```python
from build123d import *

# Parameters (mm, degrees)
SKETCH_R      = 6
SKETCH_R_2    = 3.4
PAD_DEPTH     = 8
SKETCH001_R   = 8.8
SKETCH001_R_2 = 3.4
PAD001_DEPTH  = 1
SKETCH002_R   = 4.2
SKETCH002_R_2 = 3.4
PAD002_DEPTH  = 8
FILLET_R      = 4.4


with BuildPart() as part:
    # Sketch → Pad (new body)
    with BuildSketch(Plane.XY):
        Circle(SKETCH_R)
        Circle(SKETCH_R_2, mode=Mode.SUBTRACT)
    extrude(amount=PAD_DEPTH)

    # Sketch001 → Pad001 (new body)
    with BuildSketch(Plane.XY.offset(8)):
        Circle(SKETCH001_R)
        Circle(SKETCH001_R_2, mode=Mode.SUBTRACT)
    extrude(amount=PAD001_DEPTH)

    # Sketch002 → Pad002 (new body)
    with BuildSketch(Plane.XY.offset(9)):
        Circle(SKETCH002_R)
        Circle(SKETCH002_R_2, mode=Mode.SUBTRACT)
    extrude(amount=PAD002_DEPTH)

    # Fillet
    fillet_edges = [part.edges().sort_by_distance(p)[0] for p in [
        (-4.2, 0, 9),
    ]]
    fillet(fillet_edges, radius=FILLET_R)


solid = part.part
```
Check sheet for the modelled part. Datum: model origin and axes. Units: mm. A direction names the side the tool comes from. Coordinates: 2 decimals unless noted, no trailing zeros. Loops run counter-clockwise (first coordinate to the right, second up) from the corner with the lowest first, then second, coordinate; pieces in that order, holes last. Notation, with made-up numbers: M -4,35 L 37,35 A19 cw 37,61 Z; hole C 14.5,51 d4. An arc over 180 degrees is marked long. Answer as a JSON object with one key per item and string values.
1. Scan lines: L1, parallel to Y at x = 0, z = 7.75; L2, parallel to Y at x = 0, z = 10.25; L3, parallel to X at y = -0.25, z = 10.75. Record each from-to range of solid material in increasing order. Write a range as from..to.
Outcome:
{"L1": "-6..-3.4, 3.4..6", "L2": "-5.53..-3.4, 3.4..5.53", "L3": "-5.08..-3.39, 3.39..5.08"}
2. Sectioned sample at C-C on z = 9.25. Record the cut outline in (x, y), and give its area (3 significant figures).
Outcome:
{"outline": "C 0,0 d14.28; hole C 0,0 d6.8", "area": "124 mm²"}
3. Release check for a two-part mould opening along Y. For faces 4 (the cylindrical face through (-0.74, -3.32, 8.38)), 5 (the cylindrical face through (-6, 0, 4)), 6 (the flat face through (3, -3, 0)) record: pulls with the +Y half, pulls with the -Y half, needs draft (parallel to the pull), parting line crosses it, or undercut.
Outcome:
{"face 4": "undercut", "face 5": "parting line crosses it", "face 6": "needs draft"}
4. Depth check by flat-ended pin: P1, Ø1, axis at y = 5, z = 6, coming from the +X side; P2, Ø1, axis at x = 0.5, z = 1.5, coming from the +Y side; P3, Ø2, axis at y = 3, z = 12.5, coming from the -X side. Enter the tip coordinate at first touch or a pass-through.
Outcome:
{"P1": "x = 3.97", "P2": "y = 6", "P3": "x = -3.88"}
5. Sectioned sample at A-A on x = 0. Record the cut outline in (y, z), and give its area (3 significant figures).
Outcome:
{"outline": "M -8.8,8 L -6,8 L -6,0 L -3.4,0 L -3.4,17 L -4.2,17 L -4.2,13.4 A4.4 cw -8.6,9 L -8.8,9 Z; M 3.4,0 L 6,0 L 6,8 L 8.8,8 L 8.8,9 L 8.6,9 A4.4 cw 4.2,13.4 L 4.2,17 L 3.4,17 Z", "area": "73.5 mm²"}
6. Sectioned sample at D-D on z = 12. Record the cut outline in (x, y).
Outcome:
{"outline": "C 0,0 d8.86; hole C 0,0 d6.8"}
7. Access from +Z, -Z, +X, -X, +Y, -Y to the whole of each face (thin tool, end or side, straight path). Record for faces 1 (the flat face through (2, -3, 17)), 2 (the cylindrical face through (4.006, 1.262, 15.175)), 3 (the flat face through (2, -6, 8)).
Outcome:
{"face 1": "+Z, +X, -X, +Y, -Y", "face 2": "+Z", "face 3": "-Z"}
